from build123d import *

# Parameters (mm, degrees)
F0_R        = 14.25831
F0_R_2      = 22.469568
F1_DEPTH    = 6.858
F1_FACE_R   = 14.25831
F1_FACE_R_2 = 22.469568
F3_DEPTH    = 51.562


with BuildPart() as f1:
    # F0 (on Front) → F1 (new body)
    with BuildSketch(Plane.XZ):
        with BuildLine():
            Line((-12.215332, 47.053497), (-52.917511, 34.734328))
            ThreePointArc((-52.917511, 34.734328), (-82.304308, 14.977358), (-48.153338, 24.338603))
            Line((-48.153338, 24.338603), (-10.768532, 35.653716))
            ThreePointArc((-10.768532, 35.653716), (47.15239, 48.796433), (-12.215332, 47.053497))
        make_face()
        with Locations((-65.994643, 22.451784)):
            Circle(F0_R, mode=Mode.SUBTRACT)
        with Locations((17.553231, 45.039865)):
            Circle(F0_R_2, mode=Mode.SUBTRACT)
    extrude(amount=F1_DEPTH)

    # F2 (on Front) + F1_face (on face) → F3 (cut)
    with BuildSketch(Plane.XZ):
        with BuildLine():
            Line((-17.678859, 42.090312), (-47.776841, 33.02855))
            ThreePointArc((-47.776841, 33.02855), (-50.269829, 29.278588), (-45.835037, 28.497672))
            Line((-45.835037, 28.497672), (-15.089784, 37.883066))
            ThreePointArc((-15.089784, 37.883066), (-13.809394, 41.571259), (-17.678859, 42.090312))
        make_face()
    with BuildSketch(Plane(origin=(-8.49041, -6.858, 38.801754), x_dir=(1, 0, 0), z_dir=(0, -1, 0))):
        with BuildLine():
            Line((-39.662928, -14.46315), (-2.278122, -3.148038))
            ThreePointArc((-2.278122, -3.148038), (55.6428, 9.99468), (-3.724922, 8.251743))
            Line((-3.724922, 8.251743), (-44.427102, -4.067426))
            ThreePointArc((-44.427102, -4.067426), (-73.813899, -23.824395), (-39.662928, -14.46315))
        make_face()
        with Locations((-57.504233, -16.349969)):
            Circle(F1_FACE_R, mode=Mode.SUBTRACT)
        with Locations((26.043641, 6.238111)):
            Circle(F1_FACE_R_2, mode=Mode.SUBTRACT)
    extrude(amount=F3_DEPTH, mode=Mode.SUBTRACT)


solid = f1.part
Part model, mm, in its own coordinate system. A direction names the side the tool comes from. Give positions to 0.01 mm unless a question says otherwise; leave off trailing zeros. Loops run counter-clockwise (first coordinate to the right, second up) from the corner with the lowest first, then second, coordinate; pieces in that order, holes last. Notation, with made-up numbers: (36, 74.25) -> (80, 74.25) arc R26 cw to (80, 94.25) -> close; hole circle Ø6 at (21, 89.5). An arc over 180 degrees is marked (long way). Write each question's results on one line, items separated by ' | '. Start each with the question number.
Q1. Pin check, flat tips, straight feed: P1, Ø2, axis at x = -32, y = -1, coming from the -Z side (3 decimals); P2, Ø1, axis at x = 24, y = -2, coming from the +Z side; P3, Ø1.5, axis at x = -47.5, y = -1, coming from the +Z side. Stop position of each tip, or through.
Q2. Wall check: L1, parallel to X at y = -4, z = 22; L2, parallel to X at y = -1, z = 9.5; L3, parallel to Z at x = 7, y = -3.75. Give the ranges that are in metal, low to high.
Q3. Band-saw the part on D-D on z = 17. List the corners of the cut face in (x, y).
Q4. Band-saw the part on C-C on y = -4.25. List the corners of the cut face in (x, z), plus the area to 3 significant figures.
Q5. Pull direction Z, two halves, no side cores. Call faces 4 (the face through (38.309, -3.381, 36.434)), 5 (the face through (-9, 0, 40)), 6 (the face through (47.282, -3.381, 47.572)): +Z half, -Z half, draft (parallel to the pull), parting line (faces both ways), or undercut.
Q6. Band-saw the part on A-A on z = 50.5. List the corners of the cut face in (x, y), plus the area to 3 significant figures.
Q7. Band-saw the part on B-B on x = -65.5. List the corners of the cut face in (y, z).
Q8. Which spindle directions (+Z, -Z, +X, -X, +Y, -Y) get a long thin tool onto all of the face, cutting with end or side? Do faces 1 (the face through (-32.28, -3.38, 40.98)), 2 (the face through (-9, -6.858, 40)), 3 (the face through (-30.678, -3.381, 33.125)). Say none if no direction does.
Results are:
1) P1: stops at z = 28.925 | P2: stops at z = 74.28 | P3: stops at z = 36.6
2) L1: x = -83.93 to -80.25, -51.74 to -48.06, -1.4 to 36.51 | L2: x = -78.41 to -71.96, -60.03 to -53.58 | L3: z = 17.13 to 25.2, 64.88 to 72.95
3) outline: (-83.09, -6.86) -> (-79.17, -6.86) -> (-79.17, 0) -> (-83.09, 0) -> close; (-52.82, -6.86) -> (-48.9, -6.86) -> (-48.9, 0) -> (-52.82, 0) -> close; (7.36, -6.86) -> (27.75, -6.86) -> (27.75, 0) -> (7.36, 0) -> close
4) outline: (-52.92, 34.73) arc R17.94 ccw (long way) to (-48.15, 24.34) -> (-10.77, 35.65) arc R29.84 ccw (long way) to (-12.22, 47.05) -> close; hole circle Ø28.52 at (-65.99, 22.45); hole (-47.78, 33.03) arc R2.69 ccw (long way) to (-45.84, 28.5) -> (-15.09, 37.88) arc R2.52 ccw (long way) to (-17.68, 42.09) -> close; hole circle Ø44.94 at (17.55, 45.04) | area: 1,850 mm²
5) face 4: undercut | face 5: draft | face 6: parting line
6) outline: (-11.78, -6.86) -> (-4.24, -6.86) -> (-4.24, 0) -> (-11.78, 0) -> close; (39.35, -6.86) -> (46.89, -6.86) -> (46.89, 0) -> (39.35, 0) -> close | area: 103 mm²
7) outline: (-6.86, 4.52) -> (0, 4.52) -> (0, 8.2) -> (-6.86, 8.2) -> close; (-6.86, 36.7) -> (0, 36.7) -> (0, 40.39) -> (-6.86, 40.39) -> close
8) face 1: +Z, +Y, -Y | face 2: +Z, -Z, +X, -X, -Y | face 3: +Y, -Y
